Autodesk Inventor part; units mm, degrees
ref_plane "YZ Plane" through (0, 0, 0) normal (1, 0, 0) x (0, 1, 0)
ref_plane "XZ Plane" through (0, 0, 0) normal (0, 1, 0) x (-1, 0, 0)
ref_plane "XY Plane" through (0, 0, 0) normal (0, 0, 1) x (1, 0, 0)
sketch "Sketch1" plane through (0, 0, 0) normal (0, 0, 1) x (1, 0, 0)
  line L0 (0, 0) -> (-25.4, 0)
  line L1 (-25.4, 0) -> (-406.4, 203.2)
  line L2 (-406.4, 203.2) -> (-457.2, 203.2)
  line L3 (-457.2, 203.2) -> (-457.2, 206.1972)
  line L4 (-457.2, 206.1972) -> (-405.6507, 206.1972)
  line L5 (-405.6507, 206.1972) -> (-24.6507, 2.9972)
  line L6 (-24.6507, 2.9972) -> (0, 2.9972)
  line L7 (0, 2.9972) -> (0, 0)
  line L8 (-406.4, 203.2) -> (-405.6507, 206.1972) construction
  line L9 (-24.6507, 2.9972) -> (-25.4, 0) construction
  line L10 (0, 0) -> (-457.2, 0) construction
  line L11 (-457.2, 0) -> (-457.2, 206.1972) construction
  line L12 (-457.2, 206.1972) -> (0, 206.1972) construction
  line L13 (0, 206.1972) -> (0, 0) construction
  line L14 (-406.4, 203.2) -> (-449.1958, 32.0169) construction
  dimension "d0" = 2.9972
  dimension "d1" = 2.9972
  dimension "d2" = 381
  dimension "d3" = 203.2
  dimension "d5" = 50.8
  dimension "d6" = 25.4
  dimension "d7" = 151.928
extrude "Extrusion1" add sketch "Sketch1" along normal blind 558.8
sketch "Sketch2" plane through (0, 0, 558.8) normal (0, 0, 1) x (1, 0, 0)
  line L0 (-25.4, 0) -> (0, 0)
  line L1 (0, 0) -> (-25.4, 0)
  line L2 (-457.2, 203.2) -> (-406.4, 203.2)
  line L3 (-25.4, 0) -> (-406.4, 203.2)
  line L4 (-406.4, 203.2) -> (-457.2, 203.2)
  line L5 (-457.2, 206.1972) -> (-457.2, 203.2)
  line L6 (-457.2, 203.2) -> (-457.2, 206.1972)
  line L7 (-24.6507, 2.9972) -> (-405.6507, 206.1972)
  line L8 (-457.2, 206.1972) -> (-405.6507, 206.1972)
  line L9 (-405.6507, 206.1972) -> (-24.6507, 2.9972)
  line L10 (-24.6507, 2.9972) -> (0, 2.9972)
  line L11 (0, 2.9972) -> (0, 0)
extrude "Extrusion2" cut sketch "Sketch2" against normal blind 50.8
sketch "Sketch3" plane through (0, 0, 0) normal (0, 0, -1) x (-1, 0, 0)
  line L0 (406.4, 203.2) -> (25.4, 0)
  line L1 (0, 0) -> (25.4, 0)
  line L2 (25.4, 0) -> (406.4, 203.2)
  line L3 (457.2, 203.2) -> (406.4, 203.2)
  line L4 (406.4, 203.2) -> (457.2, 203.2)
  line L5 (457.2, 206.1972) -> (457.2, 203.2)
  line L6 (457.2, 203.2) -> (457.2, 206.1972)
  line L7 (405.6507, 206.1972) -> (457.2, 206.1972)
  line L8 (457.2, 206.1972) -> (405.6507, 206.1972)
  line L9 (24.6507, 2.9972) -> (405.6507, 206.1972)
  line L10 (405.6507, 206.1972) -> (24.6507, 2.9972)
  line L11 (0, 2.9972) -> (24.6507, 2.9972)
  line L12 (24.6507, 2.9972) -> (0, 2.9972)
  line L13 (0, 0) -> (0, 2.9972)
  line L14 (0, 2.9972) -> (0, 0)
extrude "Extrusion3" cut sketch "Sketch3" against normal blind 50.8
properties part number "Bottom Lexan Shield for Balls" material "Polycarbonate, Clear"
Input: part model. Units: mm. Frame: model coordinates. A direction names the side the tool comes from. Coordinates: 2 decimals unless noted, no trailing zeros. Loops run counter-clockwise (first coordinate to the right, second up) from the corner with the lowest first, then second, coordinate; pieces in that order, holes last. Notation, with made-up numbers: M 84.5,-16.5 L 129.5,-16.5 A22 cw 129.5,-1.5 Z; hole C -37.75,78 d1. An arc over 180 degrees is marked long. Use a Markdown table: item, result. Add a question column.
1) Draft query along X for faces 1 (the flat face through (-432, 206.197, 276)), 2 (the flat face through (-213.233, 100.178, 276.2)), 3 (the flat face through (-217.82, 106.02, 276.2)). Return one class per face: +X half, -X half, draft (parallel to the pull), parting line (faces both ways), or undercut.
2) Section A-A, the plane z = 436.5. Return the cut outline in (x, y).
3) Section B-B, the plane x = -412.5. Return the cut outline in (y, z).
4) Line query: L1, parallel to X at y = 89.5, z = 188; L2, parallel to X at y = 179, z = 291 (3 decimals); L3, parallel to Y at x = -47, z = 186. Output: solid intervals per line, ascending. Write a range as from..to.
5) Set-up query: faces 4 (the flat face through (-13, 0, 276)), 5 (the flat face through (-431, 203.2, 276)), 6 (the flat face through (-12, 2.997, 276)). Return all of +Z, -Z, +X, -X, +Y, -Y with unobstructed straight access to the full face (end or side cutting, diameter ignored); none if empty.
6) Pin query (flat end, axial travel): P1, Ø3, axis at x = -216, z = 211, coming from the +Y side; P2, Ø5, axis at x = -311.5, z = 152.5, coming from the +Y side; P3, Ø3, axis at y = 31, z = 450, coming from the -X side. Return the tip coordinate at first contact, or that it passes through.
7) Section C-C, the plane y = 35. Return the cut outline in (x, z) (3 decimals), plus the area to 3 significant figures.
Answer below:
| question | item | result |
|---|---|---|
| 1 | face 1 | draft |
| 1 | face 2 | -X half |
| 1 | face 3 | +X half |
| 2 | outline | M -457.2,203.2 L -406.4,203.2 L -25.4,0 L 0,0 L 0,3 L -24.65,3 L -405.65,206.2 L -457.2,206.2 Z |
| 3 | outline | M 203.2,50.8 L 206.2,50.8 L 206.2,508 L 203.2,508 Z |
| 4 | L1 | -193.21..-186.84 |
| 4 | L2 | -361.025..-354.656 |
| 4 | L3 | 11.52..14.92 |
| 5 | face 4 | +Z, -Z, +X, -X, -Y |
| 5 | face 5 | +Z, -Z, -X, -Y |
| 5 | face 6 | +Z, -Z, +X, +Y |
| 6 | P1 | y = 105.85 |
| 6 | P2 | y = 157.32 |
| 6 | P3 | x = -86.34 |
| 7 | outline | M -91.025,50.8 L -84.656,50.8 L -84.656,508 L -91.025,508 Z |
| 7 | area | 2,910 mm2 |
